CAD build for the part. Positions are in the model's coordinates, mm. A direction names the side the tool comes from. Give positions to 0.01 mm unless a question says otherwise; leave off trailing zeros. Write each loop counter-clockwise with the first axis right and the second up, starting at its lowest first coordinate (ties: lowest second). Pieces come first, ordered by that corner, then holes. Notation, with made-up numbers: (75, 34.5) -> (102, 34.5) arc R20 ccw to (102, 50.5) -> close; hole circle Ø7 at (18, 34.5). An arc over 180 degrees is marked (long way). Answer as a JSON object with one key per item and string values.
```python
from build123d import *

# Parameters (mm, degrees)
CIRPATTERN1_COUNT = 4


with BuildPart() as part:
    # Sketch1 → Revolve1 (revolve)
    with BuildSketch(Plane(origin=(0, 0, 0), x_dir=(0, 0, -1), z_dir=(1, 0, 0))):
        with BuildLine():
            Line((-4.43484, 0), (1.61544, 0))
            Line((1.61544, 0), (1.61544, 3.2258))
            Line((1.61544, 3.2258), (6.05028, 3.2258))
            Line((6.05028, 3.2258), (6.05028, 8.45566))
            Line((6.05028, 8.45566), (3.62966, 8.45566))
            Line((3.62966, 8.45566), (3.62966, 9.6647))
            Line((3.62966, 9.6647), (-3.62966, 9.6647))
            Line((-3.62966, 9.6647), (-3.62966, 8.45566))
            Line((-3.62966, 8.45566), (-6.05028, 8.45566))
            Line((-6.05028, 8.45566), (-6.05028, 6.03504))
            Line((-6.05028, 6.03504), (-2.82448, 6.03504))
            Line((-2.82448, 6.03504), (-2.82448, 2.792156737))
            ThreePointArc((-2.82448, 2.792156737), (-4.003397886, 1.6116295), (-4.43484, 0))
        make_face()
    revolve(axis=Axis((0, 0, 4.43484), (0, 0, -1)))

    # Sketch2 → Cut-Revolve1 (revolve, cut)
    with BuildSketch(Plane.XY.offset(2.82448)):
        with BuildLine():
            Line((-1.20904, 4.318), (1.20904, 4.318))
            ThreePointArc((1.20904, 4.318), (0, 5.52704), (-1.20904, 4.318))
        make_face()
    cut_revolve1 = revolve(axis=Axis((-1.20904, 4.318, 2.82448), (1, 0, 0)), mode=Mode.SUBTRACT)

    # CirPattern1: Cut-Revolve1 ×4 about axis
    cirpattern1_axis = Axis((0, 0, 0), (0, 0, 1))
    for i in range(1, CIRPATTERN1_COUNT):
        add(cut_revolve1.rotate(cirpattern1_axis, i * 360 / CIRPATTERN1_COUNT), mode=Mode.SUBTRACT)


solid = part.part
```
1) Slice it at D-D (y = 2.5). List the corners of the cut face in (x, z).
Model answer:
{"outline": "(-9.34, -3.63) -> (-8.08, -3.63) -> (-8.08, -6.05) -> (-2.04, -6.05) -> (-2.04, -1.62) -> (2.04, -1.62) -> (2.04, -6.05) -> (8.08, -6.05) -> (8.08, -3.63) -> (9.34, -3.63) -> (9.34, 3.63) -> (8.08, 3.63) -> (8.08, 6.05) -> (5.49, 6.05) -> (5.49, 2.82) -> (1.24, 2.82) arc R2.04 ccw to (-1.24, 2.82) -> (-5.49, 2.82) -> (-5.49, 6.05) -> (-8.08, 6.05) -> (-8.08, 3.63) -> (-9.34, 3.63) -> close"}
2) Mould opens along X. For faces 4 (the flat face through (-9, 0, -3.63)), 5 (the cylindrical face through (2.54, 8.065, -4.823)), 6 (the cylindrical face through (5.984, -0.786, 4.415)), 7 (the flat face through (0, 0, -1.615)) say: released by +X, released by -X, zero draft, split by the parting line, or undercut.
Model answer:
{"face 4": "zero draft", "face 5": "split by the parting line", "face 6": "undercut", "face 7": "undercut"}
3) Pin check, flat tips, straight feed: pin 1 (6 mm diameter, centred on x = 2.5, y = -1, fed in from +Z); pin 2 (1.5 mm diameter, centred on y = -4, z = -1.5, fed in from -X); pin 3 (1.5 mm diameter, centred on x = 6, y = -7.5, fed in from +Z). Stop position of each tip, or through.
Model answer:
{"pin 1": "stops at z = 4.43", "pin 2": "stops at x = -9.1", "pin 3": "stops at z = 3.63"}
4) 3-axis set-ups, long thin cutter, end or side, ignore diameter. For faces 1 (the flat face through (2, -6, 6.05)), 2 (the cylindrical face through (0.969, 3.077, -3.864)), 3 (the cylindrical face through (2.54, 8.065, 4.857)): which of +Z, -Z, +X, -X, +Y, -Y reach the whole face in a straight line?
Model answer:
{"face 1": "+Z, +X, -X, +Y, -Y", "face 2": "-Z", "face 3": "+Z"}
5) Slice it at A-A (y = 0). List the corners of the cut face in (x, z), then the cut area to 3 significant figures.
Model answer:
{"outline": "(-9.66, -3.63) -> (-8.46, -3.63) -> (-8.46, -6.05) -> (-3.23, -6.05) -> (-3.23, -1.62) -> (3.23, -1.62) -> (3.23, -6.05) -> (8.46, -6.05) -> (8.46, -3.63) -> (9.66, -3.63) -> (9.66, 3.63) -> (8.46, 3.63) -> (8.46, 6.05) -> (6.04, 6.05) -> (6.04, 2.82) -> (5.53, 2.82) arc R1.21 cw to (3.11, 2.82) -> (2.79, 2.82) arc R3.23 ccw to (-2.79, 2.82) -> (-3.11, 2.82) arc R1.21 cw to (-5.53, 2.82) -> (-6.04, 2.82) -> (-6.04, 6.05) -> (-8.46, 6.05) -> (-8.46, 3.63) -> (-9.66, 3.63) -> close", "area": "156 mm2"}
6) Slice it at C-C (z = -2.25). List the corners of the cut face in (x, y).
Model answer:
{"outline": "circle Ø19.33 at (0, 0); hole circle Ø6.45 at (0, 0)"}
7) Wall check: probe 1 along X at (y, z) = (0, -4); probe 2 along X at (y, z) = (0, 5.05); probe 3 along Z at (x, y) = (1, 3.5). Give the ranges that are in metal, low to high.
Model answer:
{"probe 1": "x = -8.46 to -3.23, 3.23 to 8.46", "probe 2": "x = -8.46 to -6.04, 6.04 to 8.46", "probe 3": "z = -6.05 to 2.82"}
